from build123d import *

# Parameters (mm, degrees)
F0_W     = 18.5761749744
F0_H     = 51.8475696445
F0_R     = 11.8720680475
F1_DEPTH = 6


# Not quite as in the source:
# - ends of sketch curves that miss each other by under 0.0002 mm in the source are joined
# - a feature names something its author has since deleted; it is built from what else it names


with BuildPart() as f1:
    # F0 (on Front) → F1 (new body)
    with BuildSketch(Plane.XZ):
        with BuildLine():
            add(Edge.make_bspline(
                [(192.7526748574, -288.1484243559), (215.2837565712, -280.7484243098), (215.2837563696, -43.999011342), (215.2526721504, -42.1484243381)],
                knots=[0, 0, 0, 0, 247.0268201774, 247.0268201774, 247.0268201774, 247.0268201774], degree=3))
            Line((215.2526721504, -42.1484243381), (190.2526734349, -42.1484243613))
            Line((190.2526734349, -42.1484243613), (190.2526734349, -47.1484243613))
            Line((190.2526734349, -47.1484243613), (165.2526734349, -47.1484243613))
            Line((165.2526734349, -47.1484243613), (165.2526734349, -268.1484243613))
            Line((165.2526734349, -268.1484243613), (175.2526734349, -268.1484243613))
            Line((175.2526734349, -268.1484243613), (175.2526734349, -288.1484243613))
            Line((175.2526734349, -288.1484243613), (192.7526748574, -288.1484243559))
        make_face()
        with Locations((181.4437263322, -233.8176692815)):
            Rectangle(F0_W, F0_H, mode=Mode.SUBTRACT)
        with Locations((191.5265821529, -117.0901346)):
            Circle(F0_R, mode=Mode.SUBTRACT)
        with BuildLine():
            add(Edge.make_bspline(
                [(192.7526744386, 203.8515756413), (215.2837561649, 196.4515756336), (215.2837563665, -40.2978373342), (215.2526721504, -42.1484243381)],
                knots=[0, 0, 0, 0, 247.0268201774, 247.0268201774, 247.0268201774, 247.0268201774], degree=3))
            Line((192.7526744386, 203.8515756413), (175.2526734349, 203.8515756387))
            Line((175.2526734349, 203.8515756387), (175.2526734349, 183.8515756387))
            Line((175.2526734349, 183.8515756387), (165.2526734349, 183.8515756387))
            Line((165.2526734349, 183.8515756387), (165.2526734349, -37.1484243613))
            Line((165.2526734349, -37.1484243613), (190.2526734349, -37.1484243613))
            Line((190.2526734349, -37.1484243613), (190.2526734349, -42.1484243613))
            Line((190.2526734349, -42.1484243613), (215.2526721504, -42.1484243381))
        make_face()
        with Locations((181.4437263322, 149.5208205589)):
            Rectangle(F0_W, F0_H, mode=Mode.SUBTRACT)
        with Locations((191.5265821529, 32.7932858774)):
            Circle(F0_R, mode=Mode.SUBTRACT)
    extrude(amount=F1_DEPTH)


solid = f1.part
The model under review builds one solid part; all positions refer to its coordinate system, in mm. Give positions to 0.01 mm unless a question says otherwise; leave off trailing zeros. Write each loop counter-clockwise with the first axis right and the second up, starting at its lowest first coordinate (ties: lowest second). Pieces come first, ordered by that corner, then holes. Notation, with made-up numbers: M 68.25,-32.5 L 91.25,-32.5 A8 cw 91.25,-22.5 Z; hole C 75,9 d8. An arc over 180 degrees is marked long. One line per question, with ' | ' between items. Start each with the question number.
Item 1: We need section B-B on y = -2.25. Give the number of separate pieces and of enclosed holes in the cut face, plus the area to 3 significant figures.
Item 2: For pin 1 (1.5 mm diameter, centred on x = 170.5, z = 6, fed in from +Y); pin 2 (3 mm diameter, centred on y = -2.5, z = -280, fed in from -X); pin 3 (19 mm diameter, centred on x = 191.53, z = -117.09, fed in from -Y), all flat-tipped, find the tip position at first contact; note any pin that passes through.
Item 3: Wall thickness on line 1 (Z direction, x = 177, y = -5.25); line 2 (Z direction, x = 169, y = -5); line 3 (Z direction, x = 195, y = -0.5): over which ranges is each line inside the solid? List them lowest first. Write a range as from..to.
Item 4: Draft analysis for pull direction X (two halves, no side actions). For faces 1 (the flat face through (195, -6, -39)), 2 (the cylindrical face through (202.85, -2.96, -113.52)), 3 (the cylindrical face through (202.85, -2.96, 36.36)), state which applies: released by +X, released by -X, zero draft, split by the parting line, or undercut.
Item 5: We need section A-A on x = 185.5. Write out the cut boundary in (y, z), plus the area to 3 significant figures.
Results found:
1) separate pieces: 1 | enclosed holes: 4 | area: 18,800 mm2
2) pin 1: stops at y = 0 | pin 2: stops at x = 175.25 | pin 3: passes through
3) line 1: z = -288.15..-259.74, -207.89..-47.15, -37.15..123.6, 175.44..203.85 | line 2: z = -268.15..-47.15, -37.15..183.85 | line 3: z = -286.59..-128.44, -105.74..21.44, 44.15..202.29
4) face 1: zero draft | face 2: undercut | face 3: undercut
5) outline: M -6,-288.15 L 0,-288.15 L 0,-259.74 L -6,-259.74 Z; M -6,-207.89 L 0,-207.89 L 0,-127.32 L -6,-127.32 Z; M -6,-106.86 L 0,-106.86 L 0,-47.15 L -6,-47.15 Z; M -6,-37.15 L 0,-37.15 L 0,22.56 L -6,22.56 Z; M -6,43.02 L 0,43.02 L 0,123.6 L -6,123.6 Z; M -6,175.44 L 0,175.44 L 0,203.85 L -6,203.85 Z | area: 2,020 mm2
